For this review, take the finished solid that the model builds, in its own axes (mm). A direction names the side the tool comes from. Coordinates: 2 decimals unless noted, no trailing zeros. Write each loop counter-clockwise with the first axis right and the second up, starting at its lowest first coordinate (ties: lowest second). Pieces come first, ordered by that corner, then holes. Notation, with made-up numbers: M 72,-3 L 100,-3 A31 cw 100,28 Z; hole C 52,55 d6. An arc over 180 degrees is marked long. Return JSON: item names as keys, results as strings.
```python
from build123d import *

# Parameters (mm, degrees)
F0_R     = 9.1
F0_R_2   = 6.1
F1_DEPTH = 25
F2_R     = 13.5
F2_R_2   = 9.1
F2_R_3   = 6.1
F3_DEPTH = 25
F4_R     = 9.1
F4_R_2   = 6.1
F5_DEPTH = 25
F6_R     = 6.1
F6_R_2   = 5
F7_DEPTH = 2


with BuildPart() as f1:
    # F0 (on Front) → F1 (new body)
    with BuildSketch(Plane.XZ):
        Circle(F0_R)
        Circle(F0_R_2, mode=Mode.SUBTRACT)
    extrude(amount=F1_DEPTH)

    # F2 (on face) → F3 (join)
    with BuildSketch(Plane.XZ.offset(25)):
        Circle(F2_R)
        Circle(F2_R_2, mode=Mode.SUBTRACT)
        Circle(F2_R_2)
        Circle(F2_R_3, mode=Mode.SUBTRACT)
    extrude(amount=F3_DEPTH)

    # F4 (on face) → F5 (join)
    with BuildSketch(Plane.XZ.offset(50)):
        Circle(F4_R)
        Circle(F4_R_2, mode=Mode.SUBTRACT)
    extrude(amount=F5_DEPTH)

    # F6 (on face) → F7 (join)
    with BuildSketch(Plane(origin=(0, 0, 0), x_dir=(-1, 0, 0), z_dir=(0, 1, 0))):
        Circle(F6_R)
        Circle(F6_R_2, mode=Mode.SUBTRACT)
    extrude(amount=-F7_DEPTH)


solid = f1.part
```
1. We need section D-D (y = -36). State the section outline as (x, z) points.
Checks:
{"outline": "C 0,0 d27; hole C 0,0 d12.2"}
2. Clearance check with flat-ended pins moving along their axes: pin 1 Ø1 at (y, z) = (-59.5, 4) entering from +X; pin 2 Ø4 at (x, y) = (-8.5, -65.5) entering from -Z; pin 3 Ø6 at (y, z) = (-64, 3.5) entering from +X. State where each tip first meets the part, or that it passes through.
Checks:
{"pin 1": "x = 8.4", "pin 2": "z = -6.37", "pin 3": "x = 9.09"}
3. Wall thickness on L1, parallel to Z at x = 0, y = -51; L2, parallel to Z at x = 0, y = -29; L3, parallel to Y at x = -6.5, z = 11: over which ranges is each line inside the solid? List them lowest first. Write a range as from..to.
Checks:
{"L1": "-9.1..-6.1, 6.1..9.1", "L2": "-13.5..-6.1, 6.1..13.5", "L3": "-50..-25"}
4. We need section B-B (z = 0). State the section outline as (x, y) points, plus the area to 3 significant figures.
Checks:
{"outline": "M -13.5,-50 L -9.1,-50 L -9.1,-75 L -6.1,-75 L -6.1,-2 L -5,-2 L -5,0 L -9.1,0 L -9.1,-25 L -13.5,-25 Z; M 5,-2 L 6.1,-2 L 6.1,-75 L 9.1,-75 L 9.1,-50 L 13.5,-50 L 13.5,-25 L 9.1,-25 L 9.1,0 L 5,0 Z", "area": "674 mm2"}
5. We need section A-A (x = 0). State the section outline as (y, z) points.
Checks:
{"outline": "M -75,-9.1 L -50,-9.1 L -50,-13.5 L -25,-13.5 L -25,-9.1 L 0,-9.1 L 0,-5 L -2,-5 L -2,-6.1 L -75,-6.1 Z; M -75,6.1 L -2,6.1 L -2,5 L 0,5 L 0,9.1 L -25,9.1 L -25,13.5 L -50,13.5 L -50,9.1 L -75,9.1 Z"}
6. For faces 4 (the face through (2, -75, -6)), 5 (the face through (-1.973, -12.325, -8.884)), 6 (the face through (5, -2, 2)), list the 3-axis set-ups (+Z, -Z, +X, -X, +Y, -Y) from which the entire face can be reached by the end or side of a thin tool; tool diameter is ignored.
Checks:
{"face 4": "+Z, -Z, +X, -X, -Y", "face 5": "+Y", "face 6": "-Y"}
7. We need section C-C (y = -17.5). State the section outline as (x, z) points, plus the area to 3 significant figures.
Checks:
{"outline": "C 0,0 d18.2; hole C 0,0 d12.2", "area": "143 mm2"}
8. Draft analysis for pull direction X (two halves, no side actions). For faces 1 (the face through (-1.973, -62.325, -8.884)), 2 (the face through (-6.094, -37.989, 0.268)), 3 (the face through (-4, 0, -4)), state which applies: +X half, -X half, draft (parallel to the pull), parting line (faces both ways), or undercut.
Checks:
{"face 1": "parting line", "face 2": "undercut", "face 3": "draft"}
